from build123d import *

# Parameters (mm, degrees)
F0_R          = 1.15
F0_R_2        = 0.4
F1_DEPTH      = 6
F0_R_3        = 3
F2_DEPTH      = 12
F3_SIZE2      = 0.5773502692
F3_SIZE       = 1
F4_R          = 8
F5_DEPTH      = 25
F5_DEPTH_BACK = 25


with BuildPart() as f1:
    # F0 (on Top) → F1 (new body)
    with BuildSketch(Plane.XY):
        Circle(F0_R)
        Circle(F0_R_2, mode=Mode.SUBTRACT)
    extrude(amount=F1_DEPTH)

    # F0 (on Top) → F2 (join)
    with BuildSketch(Plane.XY):
        Circle(F0_R_3)
        Circle(F0_R, mode=Mode.SUBTRACT)
    extrude(amount=F2_DEPTH)

    # F3
    f3_edges = [f1.edges().sort_by_distance(p)[0] for p in [
        (-1.15, 0, 12),
    ]]
    f3_side = f1.faces().sort_by_distance((-1.15, 0, 9))[0]
    chamfer(f3_edges, length=F3_SIZE, length2=F3_SIZE2, reference=f3_side)

    # F4 (on Right) → F5 (cut, two sides)
    with BuildSketch(Plane.YZ) as f5_sk:
        with Locations((10, 6)):
            Circle(F4_R)
        with Locations((-10, 6)):
            Circle(F4_R)
    extrude(amount=-F5_DEPTH, mode=Mode.SUBTRACT)
    extrude(f5_sk.sketch, amount=F5_DEPTH_BACK, mode=Mode.SUBTRACT)


solid = f1.part
For this review, take the finished solid that the model builds, in its own axes (mm). Give positions to 0.01 mm unless a question says otherwise; leave off trailing zeros. Loops run counter-clockwise (first coordinate to the right, second up) from the corner with the lowest first, then second, coordinate; pieces in that order, holes last. Notation, with made-up numbers: M 47.25,-6.75 L 82.25,-6.75 A34 ccw 82.25,32.25 Z; hole C -1.75,87 d6. An arc over 180 degrees is marked long. Put each result on its own line as item: value. Start each with the question number.
(1) Wall thickness on L1, parallel to Y at x = 0, z = 2.1; L2, parallel to Y at x = -0.25, z = 1; L3, parallel to Y at x = 2, z = 9.25: over which ranges is each line inside the solid? List them lowest first.
(2) Add section C-C, the plane z = 5.75. Write out the cut boundary in (x, y), then the cut area to 3 significant figures.
(3) Add section B-B, the plane z = 7.5. Write out the cut boundary in (x, y), then the cut area to 3 significant figures.
(4) For pin 1 (1 mm diameter, centred on x = 2, z = 5.5, fed in from +Y); pin 2 (1.5 mm diameter, centred on x = -2, z = 8.5, fed in from -Y), all flat-tipped, find the tip position at first contact; note any pin that passes through.
(5) The part is to be moulded in two halves that separate along X. For faces 1 (the cylindrical face through (-0.91, -0.7, 8.46)), 2 (the flat face through (0.24, -0.5, 6)), 3 (the cylindrical face through (-3, 0, 6)), 4 (the cylindrical face through (0, 2, 6)), say which applies: +X half, -X half, draft (parallel to the pull), parting line (faces both ways), or undercut.
(6) Add section A-A, the plane y = 0. Write out the cut boundary in (x, z).
Result:
1. L1: y = -3 to -0.4, 0.4 to 3
1. L2: y = -2.99 to -0.31, 0.31 to 2.99
1. L3: y = -2.24 to 2.24
2. outline: M -2.23,-2 L 2.23,-2 A3 ccw 2.23,2 L -2.23,2 A3 ccw Z; hole C 0,0 d0.8
2. area: 21.6 mm^2
3. outline: M -2.1,-2.14 L 2.1,-2.14 A3 ccw 2.1,2.14 L -2.1,2.14 A3 ccw Z; hole C 0,0 d2.3
3. area: 19.2 mm^2
4. pin 1: stops at y = 2.06
4. pin 2: stops at y = -2.6
5. face 1: undercut
5. face 2: undercut
5. face 3: parting line
5. face 4: draft
6. outline: M -3,0 L -0.4,0 L -0.4,6 L -1.15,6 L -1.15,11 L -1.73,12 L -3,12 Z; M 0.4,0 L 3,0 L 3,12 L 1.73,12 L 1.15,11 L 1.15,6 L 0.4,6 Z
